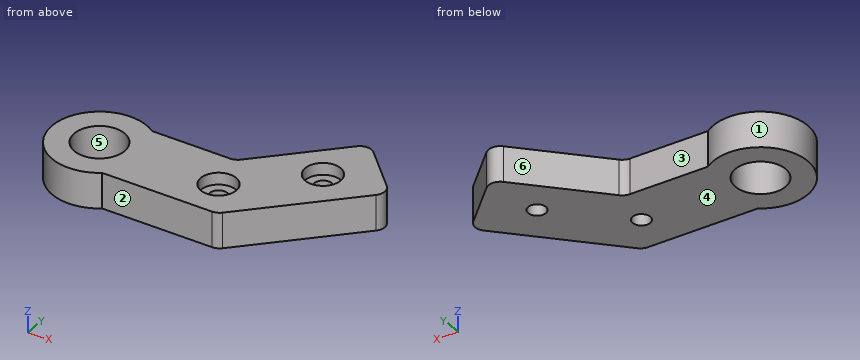
```python
from build123d import *

# Parameters (mm, degrees)
BOSS_EXTRU_1_DEPTH      = 6
CONG_1_R                = 2
ESQUISSE2_R             = 4.25
ESQUISSE2_R_2           = 1.5
ENL_V_MAT_EXTRU_1_DEPTH = 36.335346375
ESQUISSE3_R             = 3
ENL_V_MAT_EXTRU_2_DEPTH = 2


with BuildPart() as part:
    # Esquisse1 → Boss.-Extru.1 (new body)
    with BuildSketch(Plane.XY):
        with BuildLine():
            Line((-16.712083242, 5.657318013), (-2.712083242, 5.657318013))
            Line((-2.712083242, 5.657318013), (11.157974444, 19.527375698))
            Line((11.157974444, 19.527375698), (20.350362599, 10.334987543))
            Line((20.350362599, 10.334987543), (2.672693069, -7.342681987))
            Line((2.672693069, -7.342681987), (-16.712083242, -7.342681987))
            ThreePointArc((-16.712083242, -7.342681987), (-29.375772768, -0.842681987), (-16.712083242, 5.657318013))
        make_face()
    extrude(amount=BOSS_EXTRU_1_DEPTH)

    # Congé1
    cong_1_edges = [part.edges().sort_by_distance(p)[0] for p in [
        (-2.712083242, 5.657318013, 3),
        (11.157974444, 19.527375698, 3),
        (20.350362599, 10.334987543, 3),
        (2.672693069, -7.342681987, 3),
    ]]
    fillet(cong_1_edges, radius=CONG_1_R)

    # Esquisse2 → Enlèv. mat.-Extru.1 (cut, through all)
    with BuildSketch(Plane.XY.offset(6)):
        with Locations((-21.375772768, -0.842681987)):
            Circle(ESQUISSE2_R)
        with Locations((-1.275772768, -0.842681987)):
            Circle(ESQUISSE2_R_2)
        with Locations((9.728897785, 9.350316885)):
            Circle(ESQUISSE2_R_2)
    extrude(amount=-ENL_V_MAT_EXTRU_1_DEPTH, mode=Mode.SUBTRACT)

    # Esquisse3 → Enlèv. mat.-Extru.2 (cut)
    with BuildSketch(Plane.XY.offset(6)):
        with Locations((-1.275772768, -0.842681987)):
            Circle(ESQUISSE3_R)
        with Locations((9.728897785, 9.350316885)):
            Circle(ESQUISSE3_R)
    extrude(amount=-ENL_V_MAT_EXTRU_2_DEPTH, mode=Mode.SUBTRACT)


solid = part.part
```
Could you check a few things on this model? Use its own coordinates, in mm. Face numbers are marked on the shaded views. A direction names the side the tool comes from. Coordinates: 2 decimals unless noted, no trailing zeros. Write each loop counter-clockwise with the first axis right and the second up, starting at its lowest first coordinate (ties: lowest second). Pieces come first, ordered by that corner, then holes. Notation, with made-up numbers: (77.25, 50.25) -> (136.25, 50.25) arc R24 cw to (136.25, 85.25) -> close; hole circle Ø5 at (19.25, -37). An arc over 180 degrees is marked (long way). One line per question, with ' | ' between items. Start each with the question number.
1. Will these pins go through, and if not, where does the flat tip stop? P1, Ø8, axis at x = -1.28, y = -0.84, coming from the +Z side; P2, Ø3, axis at x = 4.5, z = 1, coming from the +Y side; P3, Ø3, axis at x = 9, y = 8.5, coming from the +Z side; P4, Ø3, axis at x = 1, z = 3, coming from the +Y side.
2. If we section it at D-D (y = -3.25): Please give me the cut outline in (x, z), and give its area (3 significant figures).
3. If we section it at A-A (y = 0): Please give me the cut outline in (x, z).
4. If we section it at C-C (z = 5.35): Please give me the cut outline in (x, y), and give its area (3 significant figures).
5. For the marked faces 1, 2 and 3, which set-ups out of +Z, -Z, +X, -X, +Y, -Y let a thin tool reach every point of the face, with its end or its side?
6. Please list where these lines run through material, in increasing order: line 1 along X through (y, z) = (-1.25, 5.35); line 2 along X through (y, z) = (-1.25, 3.55); line 3 along Y through (x, z) = (-7.5, 4.3).
7. Thinking about a two-plate mould opening in Y: for the marked faces 4, 5 and 6, which applies, pulls with the +Y half, pulls with the -Y half, needs draft (parallel to the pull), parting line crosses it, or undercut?
8. If we section it at B-B (x = -20.5): Please give me the cut outline in (y, z), and give its area (3 significant figures).
Return value:
1) P1: stops at z = 6 | P2: stops at y = 14.37 | P3: stops at z = 4 | P4: stops at y = 10.87
2) outline: (-29, 0) -> (-24.88, 0) -> (-24.88, 6) -> (-29, 6) -> close; (-17.87, 0) -> (6.77, 0) -> (6.77, 6) -> (0.51, 6) -> (0.51, 4) -> (-3.07, 4) -> (-3.07, 6) -> (-17.87, 6) -> close | area: 165 mm²
3) outline: (-29.33, 0) -> (-25.54, 0) -> (-25.54, 6) -> (-29.33, 6) -> close; (-17.21, 0) -> (-2.52, 0) -> (-2.52, 4) -> (-4.15, 4) -> (-4.15, 6) -> (-17.21, 6) -> close; (-0.03, 0) -> (10.02, 0) -> (10.02, 6) -> (1.6, 6) -> (1.6, 4) -> (-0.03, 4) -> close
4) outline: (-16.71, -7.34) -> (1.84, -7.34) arc R2 ccw to (3.26, -6.76) -> (18.94, 8.92) arc R2 ccw to (18.94, 11.75) -> (12.57, 18.11) arc R2 ccw to (9.74, 18.11) -> (-2.13, 6.24) arc R2 cw to (-3.54, 5.66) -> (-16.71, 5.66) arc R8 ccw (long way) to start; hole circle Ø8.5 at (-21.38, -0.84); hole circle Ø6 at (-1.28, -0.84); hole circle Ø6 at (9.73, 9.35) | area: 563 mm²
5) face 1: +Z, -Z | face 2: +Z, -Z, +X, -Y | face 3: +Z, -Z, +Y
6) line 1: x = -29.37 to -25.61, -17.15 to -4.25, 1.7 to 8.77 | line 2: x = -29.37 to -25.61, -17.15 to -2.72, 0.17 to 8.77 | line 3: y = -7.34 to 5.66
7) face 4: needs draft | face 5: undercut | face 6: pulls with the +Y half
8) outline: (-8.79, 0) -> (-5, 0) -> (-5, 6) -> (-8.79, 6) -> close; (3.32, 0) -> (7.11, 0) -> (7.11, 6) -> (3.32, 6) -> close | area: 45.5 mm²
